Work out the finished part from the listing and answer in its coordinate system (mm). Face numbers are marked on the shaded views. Coordinates: 2 decimals unless noted, no trailing zeros. Loops run counter-clockwise (first coordinate to the right, second up) from the corner with the lowest first, then second, coordinate; pieces in that order, holes last.
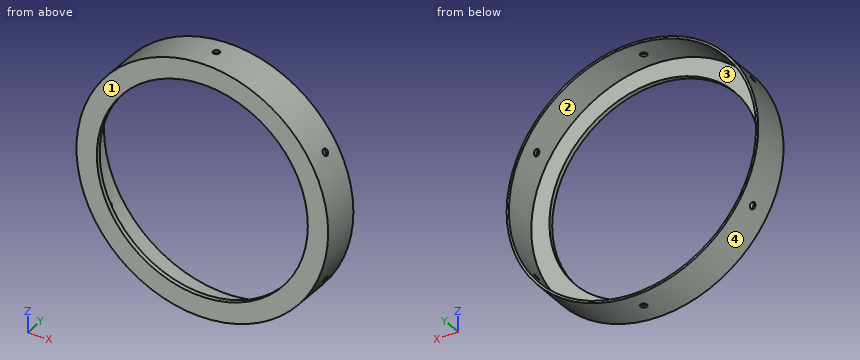
```python
from build123d import *

# Parameters (mm, degrees)
SKETCH1_R           = 90.884375
BOSS_EXTRUDE1_DEPTH = 28.575
SKETCH2_R           = 89.296875
CUT_EXTRUDE1_DEPTH  = 25.4
SKETCH3_R           = 76.2
CUT_EXTRUDE2_DEPTH  = 4.175
SKETCH4_R           = 2.413
CUT_EXTRUDE3_DEPTH  = 91.884375
CIRPATTERN1_COUNT   = 6


with BuildPart() as part:
    # Sketch1 → Boss-Extrude1 (new body)
    with BuildSketch(Plane(origin=(0, 0, 0), x_dir=(1, 0, 0), z_dir=(0, 1, 0))):
        Circle(SKETCH1_R)
    extrude(amount=BOSS_EXTRUDE1_DEPTH)

    # Sketch2 → Cut-Extrude1 (cut)
    with BuildSketch(Plane(origin=(0, 28.575, 0), x_dir=(1, 0, 0), z_dir=(0, 1, 0))):
        Circle(SKETCH2_R)
    extrude(amount=-CUT_EXTRUDE1_DEPTH, mode=Mode.SUBTRACT)

    # Sketch3 → Cut-Extrude2 (cut, through all)
    with BuildSketch(Plane(origin=(0, 3.175, 0), x_dir=(1, 0, 0), z_dir=(0, 1, 0))):
        Circle(SKETCH3_R)
    extrude(amount=-CUT_EXTRUDE2_DEPTH, mode=Mode.SUBTRACT)

    # Sketch4 → Cut-Extrude3 (cut, symmetric)
    with BuildSketch(Plane.XY):
        with Locations((0, 15.875)):
            Circle(SKETCH4_R)
    cut_extrude3 = extrude(amount=CUT_EXTRUDE3_DEPTH, both=True, mode=Mode.SUBTRACT)

    # CirPattern1: Cut-Extrude3 ×6 about axis
    cirpattern1_axis = Axis((0, 28.575, 0), (0, 1, 0))
    for i in range(1, CIRPATTERN1_COUNT):
        add(cut_extrude3.rotate(cirpattern1_axis, i * 360 / CIRPATTERN1_COUNT), mode=Mode.SUBTRACT)


solid = part.part
```
1. A cutting plane is placed at C-C, the plane y = 25.75. Give the vertices of the cut face in (x, z), then the cut area to 3 significant figures.
2. A cutting plane is placed at A-A, the plane z = 0. Give the vertices of the cut face in (x, y) (3 decimals), then the cut area to 3 significant figures.
3. Straight lines are drawn through the part: probe 1 along X at (y, z) = (22.5, 2); probe 2 along Z at (x, y) = (0.5, 7.5); probe 3 along Y at (x, z) = (0, -90.4) (3 decimals). For each, find the intervals that lie inside material, in ascending order.
4. A cutting plane is placed at B-B, the plane x = 0. Give the vertices of the cut face in (y, z) (3 decimals), then the cut area to 3 significant figures.
5. A cutting plane is placed at D-D, the plane x = -34. Give the vertices of the cut face in (y, z) (3 decimals), then the cut area to 3 significant figures.
6. Determine the mould class of the marked faces 1, 2, 3 and 4 for opening direction X: released by +X, released by -X, zero draft, split by the parting line, or undercut.
7. Each of these flat-tipped pins is pushed along its axis until it touches: P1, Ø5, axis at y = 9.5, z = 17, coming from the +X side; P2, Ø10, axis at y = 12, z = -16.5, coming from the +X side; P3, Ø2, axis at x = 29.5, y = 10.5, coming from the -Z side; P4, Ø6.5, axis at x = 0, y = 15.875, coming from the +Z side. Where does it stop, or does it pass through?
Answers below:
1. outline: circle Ø181.77 at (0, 0); hole circle Ø178.59 at (0, 0)
1. area: 899 mm2
2. outline: (-90.884, 0) - (-76.2, 0) - (-76.2, 3.175) - (-89.297, 3.175) - (-89.297, 28.575) - (-90.884, 28.575) - close; (76.2, 0) - (90.884, 0) - (90.884, 28.575) - (89.297, 28.575) - (89.297, 3.175) - (76.2, 3.175) - close
2. area: 174 mm2
3. probe 1: x = -90.86 to -89.27, 89.27 to 90.86
3. probe 2: z = -90.88 to -89.3, 89.3 to 90.88
3. probe 3: y = 0 to 13.462, 18.288 to 28.575
4. outline: (0, -90.884) - (13.462, -90.884) - (13.462, -89.297) - (3.175, -89.297) - (3.175, -76.2) - (0, -76.2) - close; (0, 76.2) - (3.175, 76.2) - (3.175, 89.297) - (13.462, 89.297) - (13.462, 90.884) - (0, 90.884) - close; (18.288, -90.884) - (28.575, -90.884) - (28.575, -89.297) - (18.288, -89.297) - close; (18.288, 89.297) - (28.575, 89.297) - (28.575, 90.884) - (18.288, 90.884) - close
4. area: 159 mm2
5. outline: (0, -84.285) - (28.575, -84.285) - (28.575, -82.571) - (3.175, -82.571) - (3.175, -68.194) - (0, -68.194) - close; (0, 68.194) - (3.175, 68.194) - (3.175, 82.571) - (28.575, 82.571) - (28.575, 84.285) - (0, 84.285) - close
5. area: 189 mm2
6. face 1: zero draft
6. face 2: undercut
6. face 3: undercut
6. face 4: split by the parting line
7. P1: stops at x = 89.72
7. P2: stops at x = 90.15
7. P3: stops at z = -86.3
7. P4: stops at z = 90.88
